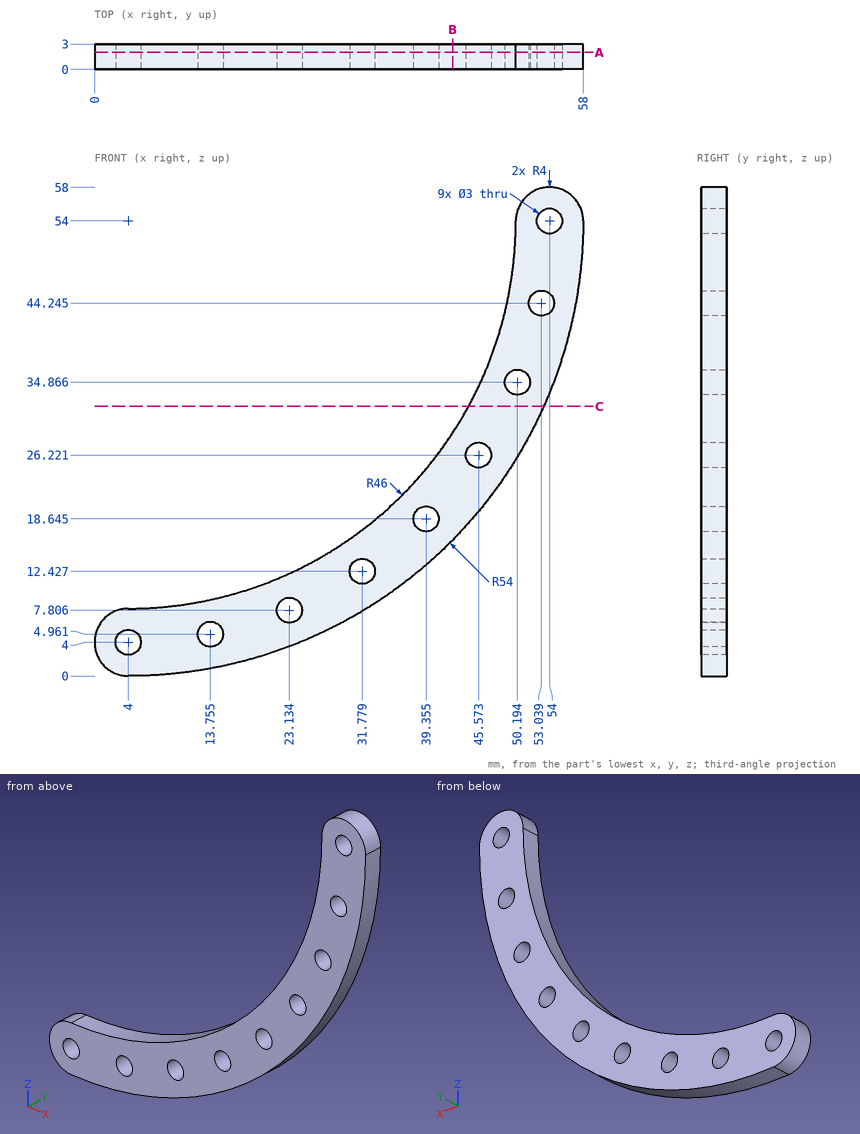
Geometry: see drawing. Coordinates: mm, zero at the bounding-box minimum. Give positions to 0.01 mm unless a question says otherwise; leave off trailing zeros. Write each loop counter-clockwise with the first axis right and the second up, starting at its lowest first coordinate (ties: lowest second). Pieces come first, ordered by that corner, then holes. Notation, with made-up numbers: M -18.75,15.25 L -0.75,15.25 A30 ccw -0.75,44.25 Z; hole C -14,5.5 d4. An arc over 180 degrees is marked long. Answer as a JSON object with one key per item and string values.
Q1. Cut plane C-C, the plane z = 32. Return the cut outline in (x, y) (1 decimal).
Geometry check:
{"outline": "M 44.4,0 L 53.3,0 L 53.3,3 L 44.4,3 Z"}
Q2. Contact query for flat-ended pins moving along their axis: P1, Ø5, axis at x = 45.57, z = 26.22, coming from the +Y side; P2, Ø1, axis at x = 35, y = 2.5, coming from the +Z side; P3, Ø1.5, axis at y = 1, z = 44.5, coming from the -X side. Output: stop coordinate, or through.
Geometry check:
{"P1": "stops at y = 3", "P2": "stops at z = 20.48", "P3": "stops at x = 48.84"}
Q3. Cut plane B-B, the plane x = 42.5. Return the cut outline in (y, z) (1 decimal).
Geometry check:
{"outline": "M 0,16.1 L 3,16.1 L 3,28.8 L 0,28.8 Z"}
Q4. Ray query, line 1 along X through (y, z) = (1, 4.5) (1 decimal); line 2 along X through (y, z) = (2.1, 45.5) (1 decimal); line 3 along Z through (x, y) = (38.5, 2.6) (1 decimal). Return the intervals inside material, ascending.
Geometry check:
{"line 1": "x = 0 to 2.6, 5.4 to 12.3, 15.2 to 25.6", "line 2": "x = 49.2 to 52.2, 53.9 to 57.3", "line 3": "z = 12.5 to 17.4, 19.9 to 23.6"}
Q5. Cut plane A-A, the plane y = 2. Count the separate pieces of the cut face and the enclosed holes in it, then the cut area to 3 significant figures.
Geometry check:
{"separate pieces": "1", "enclosed holes": "9", "area": "615 mm^2"}
